The model under review builds one solid part; all positions refer to its coordinate system, in mm. A direction names the side the tool comes from. Round coordinates to 2 decimals unless told otherwise and drop trailing zeros. Order: outer loops, then holes, each group sorted by start corner. A loop starts at its lowest first (then second) coordinate and runs counter-clockwise, first axis right, second up.
```python
from build123d import *

# Parameters (mm, degrees)
EXTRUDE_1_DEPTH          = 22
CUT_EXTRUDE_1_DEPTH      = 22
CUT_EXTRUDE_1_DEPTH_BACK = 22
SKETCH_4_R               = 5
CUT_EXTRUDE_2_DEPTH      = 22


with BuildPart() as part:
    # Sketch 1 → Extrude 1 (new body)
    with BuildSketch(Plane(origin=(0, 0, 0), x_dir=(1, 0, 0), z_dir=(0, 1, 0))):
        Polygon((0, 0), (-62, 25), (-62, -25), align=None)
    extrude(amount=EXTRUDE_1_DEPTH)

    # Sketch 3 → Cut-Extrude 1 (cut, two sides: drawn at the far end of the back side and taken through both)
    with BuildSketch(Plane.XY.offset(-CUT_EXTRUDE_1_DEPTH_BACK)):
        Polygon((-35.5, 9.009618943), (-13, 22), (-43, 22), align=None)
    extrude(amount=CUT_EXTRUDE_1_DEPTH + CUT_EXTRUDE_1_DEPTH_BACK, mode=Mode.SUBTRACT)

    # Sketch 4 → Cut-Extrude 2 (cut)
    with BuildSketch(Plane(origin=(0, 22, 0), x_dir=(1, 0, 0), z_dir=(0, 1, 0))):
        with Locations(Location((-52, -11.5, 0), (0, 0, 270))):
            Circle(SKETCH_4_R)
        with Locations(Location((-52, 11.5, 0), (0, 0, 270))):
            Circle(SKETCH_4_R)
    extrude(amount=-CUT_EXTRUDE_2_DEPTH, mode=Mode.SUBTRACT)


solid = part.part
```
(1) Insertion check: pin 1 (6 mm diameter, centred on x = -30.5, y = 4, fed in from +Z); pin 2 (6 mm diameter, centred on x = -50.5, y = 19, fed in from +Z); pin 3 (1.5 mm diameter, centred on x = -10.5, y = 14, fed in from -Z). Each pin has a flat end and moves straight along its axis. Give the tip position at first contact, or say it passes through.
Data:
pin 1: stops at z = 13.51
pin 2: stops at z = 21.57
pin 3: stops at z = -4.54
(2) For faces 1 (the flat face through (-8, 22, 0)), 2 (the flat face through (-39.302, 15.596, -0.243)), list the 3-axis set-ups (+Z, -Z, +X, -X, +Y, -Y) from which the entire face can be reached by the end or side of a thin tool; tool diameter is ignored.
Data:
face 1: +Z, -Z, +X, -X, +Y
face 2: +Z, -Z, +Y
(3) Consider section D-D (z = -2). Write out the cut boundary in (x, y).
Data:
outline: (-62, 0) - (-4.96, 0) - (-4.96, 22) - (-13, 22) - (-35.5, 9.01) - (-43, 22) - (-62, 22) - close
(4) To check wall thickness, follow probe 1 along Z at (x, y) = (-48, 11.25); probe 2 along X at (y, z) = (11.25, 11.5); probe 3 along X at (y, z) = (11.25, -7). State the ranges of each line that lie inside material, in increasing order.
Data:
probe 1: z = -19.35 to -14.5, -8.5 to 8.5, 14.5 to 19.35
probe 2: x = -62 to -57, -47 to -36.79, -31.62 to -28.52
probe 3: x = -62 to -54.18, -49.82 to -36.79, -31.62 to -17.36
(5) Consider section C-C (x = -52). Write out the cut boundary in (y, z), and give its area (3 significant figures).
Data:
outline: (0, -20.97) - (22, -20.97) - (22, -16.5) - (0, -16.5) - close; (0, -6.5) - (22, -6.5) - (22, 6.5) - (0, 6.5) - close; (0, 16.5) - (22, 16.5) - (22, 20.97) - (0, 20.97) - close
area: 483 mm2
(6) Draft analysis for pull direction X (two halves, no side actions). For faces 3 (the flat face through (-62, 11, 0)), 4 (the flat face through (-26.91, 13.97, -0.2)), 5 (the flat face through (-30.566, 10.846, -12.325)), 6 (the cylindrical face through (-47.784, 11.154, -8.812)), state which applies: pulls with the +X half, pulls with the -X half, needs draft (parallel to the pull), parting line crosses it, or undercut.
Data:
face 3: pulls with the -X half
face 4: undercut
face 5: pulls with the +X half
face 6: undercut
(7) Consider section B-B (z = 12). Write out the cut boundary in (x, y), and give its area (3 significant figures).
Data:
outline: (-62, 0) - (-56.97, 0) - (-56.97, 22) - (-62, 22) - close; (-47.03, 0) - (-29.76, 0) - (-29.76, 12.32) - (-35.5, 9.01) - (-43, 22) - (-47.03, 22) - close
area: 377 mm2
(8) Consider section A-A (y = 20.75). Write out the cut boundary in (x, z), and give its area (3 significant figures).
Data:
outline: (-62, -25) - (-42.28, -17.05) - (-42.28, 17.05) - (-62, 25) - close; (-15.17, -6.11) - (0, 0) - (-15.17, 6.11) - close; hole circle Ø10 at (-52, -11.5); hole circle Ø10 at (-52, 11.5)
area: 765 mm2
